Geometry: final body of the model. Coordinates: model frame, mm. A direction names the side the tool comes from. Give positions to 0.01 mm unless a question says otherwise; leave off trailing zeros. Write each loop counter-clockwise with the first axis right and the second up, starting at its lowest first coordinate (ties: lowest second). Pieces come first, ordered by that corner, then holes. Notation, with made-up numbers: (-20, -37) -> (7, -37) arc R31 ccw to (7, -2) -> close; hole circle Ø2 at (48, -33). An arc over 180 degrees is marked (long way). Use CSV: the item, a comma, the result in double quotes. Start each with the question number.
1) Section B-B (z = 7.25). Output: boundary loops of the cut face in (x, y) (3 decimals).
2) Material intervals for line 1 (X direction, y = 42.5, z = 10.75); line 2 (Z direction, x = 97, y = -19), sorted ascending. Write a range as [from, to].
3) Contact query for flat-ended pins moving along their axis: P1, Ø5, axis at x = 94.5, y = 19, coming from the +Z side; P2, Ø5, axis at x = -100.965, y = 61.595, coming from the -Z side; P3, Ø5.5, axis at y = 13, z = 8.5, coming from the -X side; P4, Ø4, axis at y = -26.5, z = 11, coming from the +X side. Output: stop coordinate, or through.
4) Set-up query: faces 1 (the face through (-2, -67.945, 6)), 2 (the face through (99, 1, 2)), 3 (the face through (-90, -1, 7)). Return all of +Z, -Z, +X, -X, +Y, -Y with unobstructed straight access to the full face (end or side cutting, diameter ignored); none if empty.
5) Section A-A (y = -43). Output: boundary loops of the cut face in (x, z) (3 decimals), plus the area to 3 significant figures.
```python
from build123d import *

# Parameters (mm, degrees)
SKETCH_1_W      = 214.63
SKETCH_1_H      = 135.89
SKETCH_1_R      = 1.5
EXTRUDE_1_DEPTH = 2
SKETCH_2_W      = 180
SKETCH_2_H      = 135.89
EXTRUDE_2_DEPTH = 11


with BuildPart() as part:
    # 스케치1 → 보스-돌출1 (new body)
    with BuildSketch(Plane.XY):
        Rectangle(SKETCH_1_W, SKETCH_1_H)
        with Locations((100.965, 61.595)):
            Circle(SKETCH_1_R, mode=Mode.SUBTRACT)
        with Locations((100.965, -61.595)):
            Circle(SKETCH_1_R, mode=Mode.SUBTRACT)
        with Locations(Location((-100.965, -61.595, 0), (0, 0, 180))):
            Circle(SKETCH_1_R, mode=Mode.SUBTRACT)
        with Locations(Location((-100.965, 61.595, 0), (0, 0, 180))):
            Circle(SKETCH_1_R, mode=Mode.SUBTRACT)
    extrude(amount=EXTRUDE_1_DEPTH)

    # 스케치2 → 보스-돌출2 (add)
    with BuildSketch(Plane.XY.offset(2)):
        Rectangle(SKETCH_2_W, SKETCH_2_H)
    extrude(amount=EXTRUDE_2_DEPTH)


solid = part.part
```
Answers follow:
1,outline,"(-90, -67.945) -> (90, -67.945) -> (90, 67.945) -> (-90, 67.945) -> close"
2,line 1,"x = [-90, 90]"
2,line 2,"z = [0, 2]"
3,P1,"stops at z = 2"
3,P2,"stops at z = 0"
3,P3,"stops at x = -90"
3,P4,"stops at x = 90"
4,face 1,"+Z, -Z, +X, -X, -Y"
4,face 2,"+Z, +X, +Y, -Y"
4,face 3,"+Z, -X, +Y, -Y"
5,outline,"(-107.315, 0) -> (107.315, 0) -> (107.315, 2) -> (90, 2) -> (90, 13) -> (-90, 13) -> (-90, 2) -> (-107.315, 2) -> close"
5,area,"2,410 mm^2"
